```python
from build123d import *

# Parameters (mm, degrees)
SKETCH_1_R              = 30
SKETCH_1_R_2            = 21.5
EXTRUDE_1_DEPTH         = 5
HOLE_WIZARD_3_4_3_4_1_D = 3.4
CUT_EXTRUDE_1_DEPTH     = 43.720018727


with BuildPart() as part:
    # 草图1 → 凸台-拉伸1 (new body)
    with BuildSketch(Plane.XY):
        Circle(SKETCH_1_R)
        Circle(SKETCH_1_R_2, mode=Mode.SUBTRACT)
    extrude(amount=EXTRUDE_1_DEPTH)

    # Ø3.4 (3.4) 直径孔1 (through all)
    with Locations(Plane(origin=(-25, 0, 5), x_dir=(1, 0, 0), z_dir=(0, 0, 1))):
        with Locations((0, 0), (25, 25), (25, -25), (50, 0)):
            Hole(HOLE_WIZARD_3_4_3_4_1_D / 2)

    # 草图4 → 切除-拉伸1 (cut, through all)
    with BuildSketch(Plane.XY.offset(5)):
        with BuildLine():
            Line((0, 0), (-21.213203436, 21.213203436))
            ThreePointArc((-21.213203436, 21.213203436), (0, 30), (21.213203436, 21.213203436))
            Line((21.213203436, 21.213203436), (0, 0))
        make_face()
    extrude(amount=-CUT_EXTRUDE_1_DEPTH, mode=Mode.SUBTRACT)


solid = part.part
```
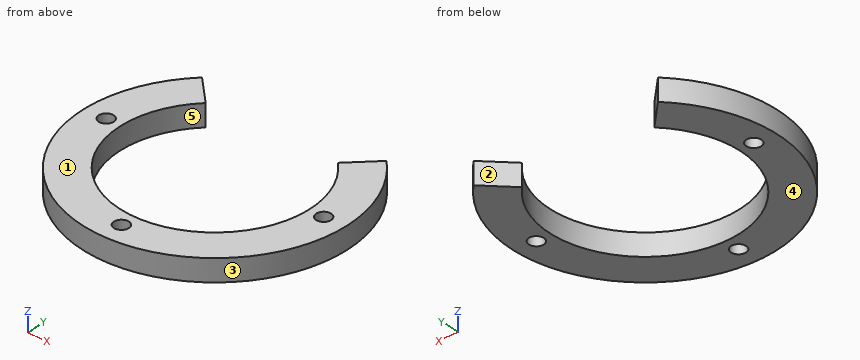
The model under review builds one solid part; all positions refer to its coordinate system, in mm. Face numbers are marked on the shaded views. A direction names the side the tool comes from. Give positions to 0.01 mm unless a question says otherwise; leave off trailing zeros. Write each loop counter-clockwise with the first axis right and the second up, starting at its lowest first coordinate (ties: lowest second). Pieces come first, ordered by that corner, then holes. Notation, with made-up numbers: (62, -29) - (109, -29) arc R17 cw to (109, 0) - close; hole circle Ø11 at (43.25, -7). An arc over 180 degrees is marked (long way). Answer in a Markdown table with one row per item. Add a question column.
1. Tool access review of the marked faces 1 and 2: name each direction out of +Z, -Z, +X, -X, +Y, -Y from which nothing blocks a thin tool from reaching the whole face with its end or side.
2. Insertion check: P1, Ø1, axis at x = -23, z = 2, coming from the -Y side; P2, Ø2, axis at y = -6.5, z = 1, coming from the -X side; P3, Ø1.5, axis at x = 16, z = 1, coming from the -Y side; P4, Ø2, axis at x = 0, y = -25, coming from the +Z side. Each pin has a flat end and moves straight along its axis. Give the tip position at first contact, or say it passes through.
3. We need section D-D on y = -6. Write out the cut boundary in (x, z).
4. Draft analysis for pull direction X (two halves, no side actions). For the marked faces 3, 4 and 5, state which applies: +X half, -X half, draft (parallel to the pull), parting line (faces both ways), or undercut.
5. We need section A-A on x = 0. Write out the cut boundary in (y, z), then the cut area to 3 significant figures.
6. We need section C-C on y = 0. Write out the cut boundary in (x, z).
7. We need section B-B on z = 4.15. Write out the cut boundary in (x, y), then the cut area to 3 significant figures.
8. Wall thickness on line 1 along X through (y, z) = (4, 0.25); line 2 along X through (y, z) = (2, 4.4); line 3 along X through (y, z) = (-23, 3.35): over which ranges is each line inside the solid? List them lowest first. Write a range as [from, to].
Ans:
| question | item | result |
|---|---|---|
| 1 | face 1 | +Z, +X, -X, +Y, -Y |
| 1 | face 2 | +Z, -Z, +Y |
| 2 | P1 | stops at y = -19.84 |
| 2 | P2 | stops at x = -29.49 |
| 2 | P3 | stops at y = -25.83 |
| 2 | P4 | passes through |
| 3 | outline | (-29.39, 0) - (-20.65, 0) - (-20.65, 5) - (-29.39, 5) - close; (20.65, 0) - (29.39, 0) - (29.39, 5) - (20.65, 5) - close |
| 4 | face 3 | parting line |
| 4 | face 4 | draft |
| 4 | face 5 | undercut |
| 5 | outline | (-30, 0) - (-26.7, 0) - (-26.7, 5) - (-30, 5) - close; (-23.3, 0) - (-21.5, 0) - (-21.5, 5) - (-23.3, 5) - close |
| 5 | area | 25.5 mm^2 |
| 6 | outline | (-30, 0) - (-26.7, 0) - (-26.7, 5) - (-30, 5) - close; (-23.3, 0) - (-21.5, 0) - (-21.5, 5) - (-23.3, 5) - close; (21.5, 0) - (23.3, 0) - (23.3, 5) - (21.5, 5) - close; (26.7, 0) - (30, 0) - (30, 5) - (26.7, 5) - close |
| 7 | outline | (-21.21, 21.21) arc R30 ccw (long way) to (21.21, 21.21) - (15.2, 15.2) arc R21.5 cw (long way) to (-15.2, 15.2) - close; hole circle Ø3.4 at (-25, 0); hole circle Ø3.4 at (0, -25); hole circle Ø3.4 at (25, 0) |
| 7 | area | 1,000 mm^2 |
| 8 | line 1 | x = [-29.73, -21.12], [21.12, 29.73] |
| 8 | line 2 | x = [-29.93, -21.41], [21.41, 29.93] |
| 8 | line 3 | x = [-19.26, 19.26] |
